Build history of the part. All positions in model axes, mm. A direction names the side the tool comes from. Coordinates: 2 decimals unless noted, no trailing zeros. Loops run counter-clockwise (first coordinate to the right, second up) from the corner with the lowest first, then second, coordinate; pieces in that order, holes last.
(1) Slice it at B-B (x = 3). Give the cut face in (y, z), and give its area (3 significant figures).
(2) Tool access for faces 4 (the face through (0, 47.476, 35)), 5 (the face through (1, -14, -31.935)), 6 (the face through (-8.606, -30.928, 33.777)), 7 (the face through (-10.205, 12.2, -21.8)), 8 (the face through (-10.041, -13, -17)): list every direction of +Z, -Z, +X, -X, +Y, -Y with a clear straight run to the whole face (end or side of a thin tool).
(3) Two-plate mould, pull along X, no slides. Class faces 1 (the face through (44.48, -10.84, -2.15)), 2 (the face through (0, 0, -40)), 3 (the face through (0.595, -21.003, 9.15)): pulls with the +X half, pulls with the -X half, needs draft (parallel to the pull), parting line crosses it, or undercut.
(4) Slice it at D-D (z = -33.5). Give the cut face in (x, y).
(5) Slice it at C-C (y = -18.5). Give the cut face in (x, z), and give its area (3 significant figures).
(6) Flat gauge pins, fed straight in: P1, Ø12, axis at x = 25, y = 0, coming from the +Z side; P2, Ø5, axis at x = -35.5, z = -36, coming from the -Y side; P3, Ø2, axis at y = -9, z = -18, coming from the +X side. Where does each tip first touch, or does it go through?
(7) Slice it at A-A (x = 22.5). Give the cut face in (y, z).
(8) Wall check: L1, parallel to Z at x = -36, y = -10; L2, parallel to Z at x = 40, y = 6; L3, parallel to X at y = -21.5, z = -40. Give the ranges that are in metal, low to high.
from build123d import *

# Parameters (mm, degrees)
F0_W     = 20.4098373652
F0_H     = 17.0696731657
F3_DEPTH = 50
F1_W     = 39.9590164423
F1_H     = 21.9808734953
F1_H_2   = 12.8620229661
F1_W_2   = 10.0409835577
F1_H_3   = 15.1571035385
F1_W_3   = 50
F1_H_4   = 13.4836062789
F1_H_5   = 14.8224066943
F1_H_6   = 21.6939870268
F4_DEPTH = 50
F5_DEPTH = 50


with BuildPart() as f3:
    # F0 (on Top) → F3 (new body, symmetric)
    with BuildSketch(Plane.XY):
        Polygon((-36.4268427715, 50), (-50, -50), (-11.1948736012, -50), (-7.6906718126, -24.1828542203), (5.3497580811, -24.1828542203), (11.394909583, -50), (50, -50), (35.9016373754, 50), align=None)
        with Locations((0, 8.5348365828)):
            Rectangle(F0_W, F0_H, mode=Mode.SUBTRACT)
    extrude(amount=F3_DEPTH, both=True)

    # F1 (on Front) → F4 (intersect, symmetric)
    with BuildSketch(Plane.XZ):
        with Locations((-30.0204917789, 39.0095632523)):
            Rectangle(F1_W, F1_H)
        with Locations((-30.0204917789, 21.5881150216)):
            Rectangle(F1_W, F1_H_2)
        with Locations((-5.0204917789, 39.0095632523)):
            Rectangle(F1_W_2, F1_H)
        with Locations((-30.0204917789, 7.5785517693)):
            Rectangle(F1_W, F1_H_3)
        with Locations((25, 39.0095632523)):
            Rectangle(F1_W_3, F1_H)
        with Locations((-30.0204917789, -6.7418031394)):
            Rectangle(F1_W, F1_H_4)
        with Locations((-5.0204917789, 7.5785517693)):
            Rectangle(F1_W_2, F1_H_3)
        with Locations((-30.0204917789, -20.894809626)):
            Rectangle(F1_W, F1_H_5)
        with Locations((-5.0204917789, -6.7418031394)):
            Rectangle(F1_W_2, F1_H_4)
        with Locations((25, 7.5785517693)):
            Rectangle(F1_W_3, F1_H_3)
        Polygon((-10.0409835577, -28.3060129732), (-50, -28.3060129732), (-50, -50), (0, -50), (0, -28.3060129732), align=None)
        with Locations((25, -6.7418031394)):
            Rectangle(F1_W_3, F1_H_4)
        with Locations((25, -39.1530064866)):
            Rectangle(F1_W_3, F1_H_6)
    extrude(amount=F4_DEPTH, both=True, mode=Mode.INTERSECT)

    # F2 (on Right) → F5 (intersect, symmetric)
    with BuildSketch(Plane.YZ):
        with BuildLine():
            ThreePointArc((-13.0180147375, 3.6492112836), (-21.5699932759, 12.268680348), (-12.9113338643, 20.780977398))
            Line((-12.9113338643, 20.780977398), (47.4755875766, 20.1275501))
            Line((47.4755875766, 20.1275501), (47.4755875766, 44.3933308125))
            Line((47.4755875766, 44.3933308125), (-9.7670806572, 44.3933308125))
            ThreePointArc((-9.7670806572, 44.3933308125), (-45.3037856876, 13.8358446009), (-13.0040198565, -20.1250519603))
            Line((-13.0040198565, -20.1250519603), (9.9475071912, -20.1250519603))
            ThreePointArc((9.9475071912, -20.1250519603), (13.7797693487, -25.4229853105), (13.1929796225, -31.9352820516))
            Line((13.1929796225, -31.9352820516), (9.74121131, -31.9352820516))
            Line((9.74121131, -31.9352820516), (-41.7333990335, -31.9352820516))
            Line((-41.7333990335, -31.9352820516), (-41.7333990335, -47.8897877038))
            Line((-41.7333990335, -47.8897877038), (33.7939150631, -47.8897877038))
            Line((33.7939150631, -47.8897877038), (38.5303236544, -47.8897877038))
            ThreePointArc((38.5303236544, -47.8897877038), (46.7972185844, -20.2080841435), (30.4012625826, 3.5782751947))
            Line((30.4012625826, 3.5782751947), (-13.0180147375, 3.6492112836))
        make_face()
    extrude(amount=F5_DEPTH, both=True, mode=Mode.INTERSECT)


solid = f3.part
Response values:
1. outline: (-24.18, -47.89) - (0, -47.89) - (0, -31.94) - (-24.18, -31.94) - close; (-24.18, -13.48) - (0, -13.48) - (0, 3.63) - (-13.02, 3.65) arc R8.57 cw to (-21.05, 15.16) - (-24.18, 15.16) - close; (-24.18, 28.02) - (0, 28.02) - (0, 44.39) - (-9.77, 44.39) arc R32.34 ccw to (-24.18, 42.56) - close; (17.07, -47.89) - (38.53, -47.89) arc R33.43 ccw to (47.08, -28.31) - (17.07, -28.31) - close; (17.07, -13.48) - (45, -13.48) arc R33.43 ccw to (30.4, 3.58) - (17.07, 3.6) - close; (17.07, 28.02) - (47.48, 28.02) - (47.48, 44.39) - (17.07, 44.39) - close
1. area: 2,650 mm2
2. face 4: +Z, -Z, +X, -X, +Y
2. face 5: +X, -X, -Y
2. face 6: +Z, -Z, -Y
2. face 7: +Z, -Z
2. face 8: +X, +Y, -Y
3. face 1: pulls with the +X half
3. face 2: undercut
3. face 3: needs draft
4. outline: (-48.88, -41.73) - (-10.07, -41.73) - (-7.69, -24.18) - (5.35, -24.18) - (9.46, -41.73) - (48.83, -41.73) - (36.44, 46.22) - (-36.94, 46.22) - close; hole (-10.2, 0) - (10.2, 0) - (10.2, 17.07) - (-10.2, 17.07) - close
5. outline: (-45.72, -47.89) - (45.56, -47.89) - (45.56, -31.94) - (-45.72, -31.94) - close; (-45.72, -19.65) - (-10.04, -19.65) - (-10.04, -13.48) - (45.56, -13.48) - (45.56, 5.64) - (-45.72, 5.64) - close; (-45.72, 18.79) - (-10.04, 18.79) - (-10.04, 28.02) - (45.56, 28.02) - (45.56, 44.09) - (-45.72, 44.09) - close
5. area: 5,220 mm2
6. P1: stops at z = 44.39
6. P2: stops at y = -41.73
6. P3: stops at x = -10.04
7. outline: (-45.21, 15.16) arc R32.34 ccw to (-32.64, -13.48) - (45, -13.48) arc R33.43 ccw to (30.4, 3.58) - (-13.02, 3.65) arc R8.57 cw to (-21.05, 15.16) - close; (-41.73, -47.89) - (38.53, -47.89) arc R33.43 ccw to (47.08, -28.31) - (14.1, -28.31) arc R9.33 cw to (13.19, -31.94) - (-41.73, -31.94) - close; (-41.22, 28.02) - (47.48, 28.02) - (47.48, 44.39) - (-9.77, 44.39) arc R32.34 ccw to start
8. L1: z = -47.89 to -31.94, -20.13 to 3.64, 20.75 to 44.42
8. L2: z = -47.89 to -31.94, -13.48 to 3.62, 28.02 to 44.39
8. L3: x = -46.13 to 45.98
